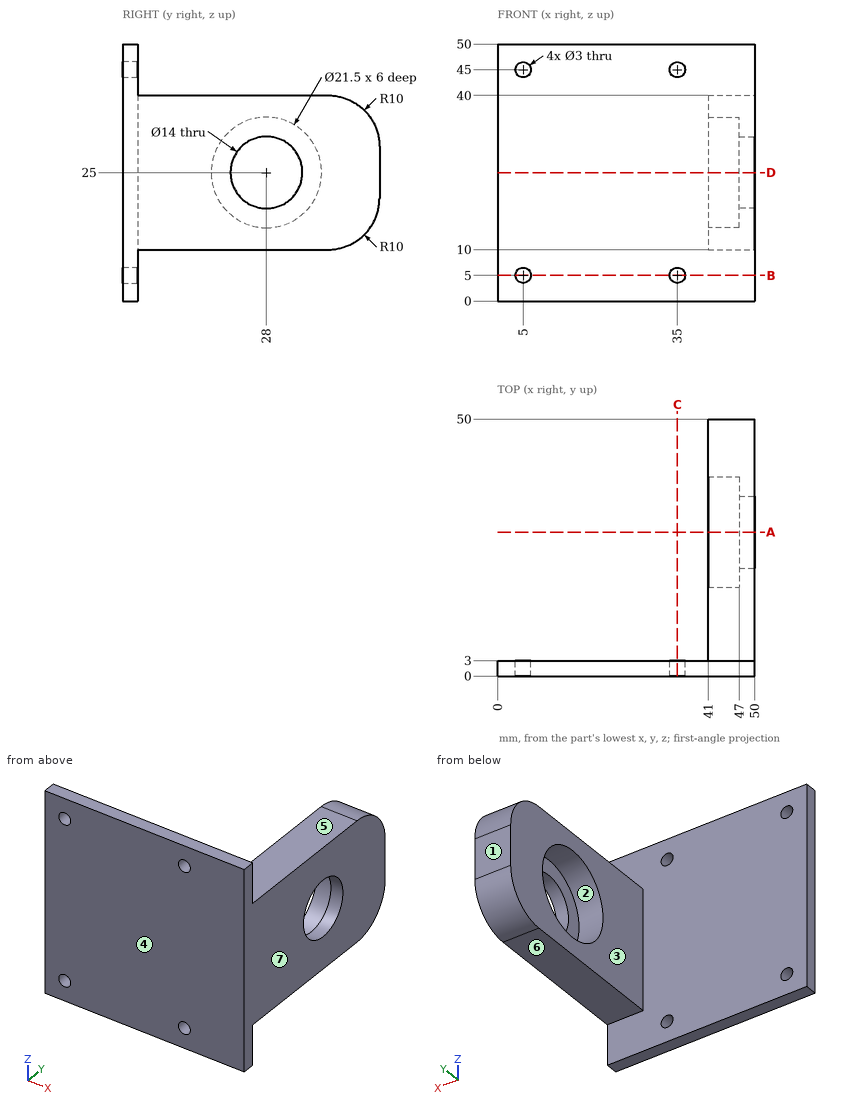
The drawing under review shows one solid part. Ordinate dimensions are in mm from its lowest x, y, z. A direction names the side the tool comes from. Round coordinates to 2 decimals unless told otherwise and drop trailing zeros. Write each loop counter-clockwise with the first axis right and the second up, starting at its lowest first coordinate (ties: lowest second). Pieces come first, ordered by that corner, then holes.
(1) We need section D-D on z = 25. Give the boundary of the cut face in (x, y), and give its area (3 significant figures).
(2) We need section A-A on y = 28. Give the boundary of the cut face in (x, z), and give its area (3 significant figures).
(3) We need section B-B on z = 5. Give the boundary of the cut face in (x, y), and give its area (3 significant figures).
(4) Machinability: for the marked faces 5, 6 and 7, which of the approach directions +Z, -Z, +X, -X, +Y, -Y give a long, thin tool a straight path to every point of the face, cutting with its end or side? Answer none if there is none.
(5) Mouldability with a two-part tool opening along Y and no side actions: class the marked faces 1, 2, 3 and 4 as +Y half, -Y half, draft (parallel to the pull), parting line (faces both ways), or undercut.
(6) Insertion check: pin 1 (10 mm diameter, centred on y = 10, z = 40, fed in from -X); pin 2 (18 mm diameter, centred on y = 28, z = 25, fed in from -X); pin 3 (8 mm diameter, centred on x = 40, y = 9, fed in from -Z); pin 4 (8 mm diameter, centred on x = 17.5, z = 30, fed in from -Y). Each pin has a flat end and moves straight along its axis. Give the tip position at first contact, or say it passes through.
(7) Wall thickness on L1, parallel to X at y = 1, z = 5; L2, parallel to Y at x = 48.25, z = 25; L3, parallel to Y at x = 10, z = 44: over which ranges is each line inside the solid? List them lowest first.
(8) We need section C-C on x = 35. Give the boundary of the cut face in (y, z), and give its area (3 significant figures).
Findings below:
1. outline: (0, 0) - (50, 0) - (50, 21) - (47, 21) - (47, 17.25) - (41, 17.25) - (41, 3) - (0, 3) - close; (41, 38.75) - (47, 38.75) - (47, 35) - (50, 35) - (50, 50) - (41, 50) - close
1. area: 402 mm2
2. outline: (41, 10) - (50, 10) - (50, 18) - (47, 18) - (47, 14.25) - (41, 14.25) - close; (41, 35.75) - (47, 35.75) - (47, 32) - (50, 32) - (50, 40) - (41, 40) - close
2. area: 99.0 mm2
3. outline: (0, 0) - (3.5, 0) - (3.5, 3) - (0, 3) - close; (6.5, 0) - (33.5, 0) - (33.5, 3) - (6.5, 3) - close; (36.5, 0) - (50, 0) - (50, 3) - (36.5, 3) - close
3. area: 132 mm2
4. face 5: +Z, +X, -X, +Y
4. face 6: -Z, +X, -X, +Y
4. face 7: +Z, -Z, +X, +Y, -Y
5. face 1: +Y half
5. face 2: undercut
5. face 3: draft
5. face 4: -Y half
6. pin 1: stops at x = 41
6. pin 2: stops at x = 47
6. pin 3: stops at z = 10
6. pin 4: stops at y = 0
7. L1: x = 0 to 3.5, 6.5 to 33.5, 36.5 to 50
7. L2: y = 0 to 21, 35 to 50
7. L3: y = 0 to 3
8. outline: (0, 0) - (3, 0) - (3, 3.5) - (0, 3.5) - close; (0, 6.5) - (3, 6.5) - (3, 43.5) - (0, 43.5) - close; (0, 46.5) - (3, 46.5) - (3, 50) - (0, 50) - close
8. area: 132 mm2
